Can you work these out from the model? Positions are in its coordinate system, mm. Round coordinates to 2 decimals unless told otherwise and drop trailing zeros. Order: outer loops, then holes, each group sorted by start corner. A loop starts at its lowest first (then second) coordinate and runs counter-clockwise, first axis right, second up. Notation, with made-up numbers: M 9,18.25 L 34,18.25 A18 ccw 34,46.25 Z; hole C 43,57 d2. An arc over 180 degrees is marked long. Answer as CSV lines item,"result". Start each with the question number.
from build123d import *

# Parameters (mm, degrees)
SKETCH10_R         = 15
CUT_EXTRUDE1_DEPTH = 31
SKETCH11_R         = 25
CUT_EXTRUDE2_DEPTH = 31


with BuildPart() as part:
    # Sketch6 → Revolve3 (revolve)
    with BuildSketch(Plane(origin=(0, 0, 0), x_dir=(1, 0, 0), z_dir=(0, 1, 0))):
        with BuildLine():
            Line((-1.369e-06, 75.786874096), (109.999998631, 75.786874096))
            ThreePointArc((109.999998631, 75.786874096), (124.999998631, 60.786874096), (109.999998631, 45.786874096))
            Line((109.999998631, 45.786874096), (-1.369e-06, 45.786874096))
            Line((-1.369e-06, 45.786874096), (-1.369e-06, 75.786874096))
        make_face()
    revolve(axis=Axis((-1.369e-06, 0, -75.786874096), (0, 0, 1)))

    # Sketch10 → Cut-Extrude1 (cut, through all)
    with BuildSketch(Plane.XY.offset(-45.786874096)):
        Circle(SKETCH10_R)
    extrude(amount=-CUT_EXTRUDE1_DEPTH, mode=Mode.SUBTRACT)

    # Sketch11 → Cut-Extrude2 (cut, through all)
    with BuildSketch(Plane.XY.offset(-45.786874096)):
        with Locations((0, 61.701118812)):
            Circle(SKETCH11_R)
        with Locations((61.701118812, 0)):
            Circle(SKETCH11_R)
        with Locations((0, -61.701118812)):
            Circle(SKETCH11_R)
        with Locations((-61.701118812, 0)):
            Circle(SKETCH11_R)
    extrude(amount=-CUT_EXTRUDE2_DEPTH, mode=Mode.SUBTRACT)


solid = part.part
(1) I want a section at C-C on x = 0. Count the separate pieces of the cut face and the enclosed holes in it, and give its area (3 significant figures).
(2) I want a section at B-B on z = -54. Write out the boundary of the cut face in (x, y).
(3) If I drill on line 1 along Y through (x, z) = (0, -60.5); line 2 along Y through (x, z) = (0, -57); line 3 along X through (y, z) = (9.5, -65.5), over which ranges is the centre line in solid material (lowest first)?
(4) I'm going to push flat-ended pins straight in: P1, Ø4, axis at y = -22.5, z = -52.5, coming from the +X side; P2, Ø1.5, axis at y = 0, z = -62.5, coming from the +X side; P3, Ø12, axis at x = 61.5, z = -67, coming from the -Y side. Where does each tip first touch, or does it pass through?
(5) I want a section at A-A on y = 0. Write out the boundary of the cut face in (x, z), and give its area (3 significant figures).
(6) If we mould it in two halves opening along Y, with no side actions, what happens to faces 1 (the cylindrical face through (-3.25, 86.49, -60.58)), 2 (the flat face through (23, 2, -45.787)), 3 (the cylindrical face through (-14.985, 0.66, -60.577))? For each: +Y half, -Y half, draft (parallel to the pull), parting line (faces both ways), or undercut.
From the geometry:
1,separate pieces,"4"
1,enclosed holes,"0"
1,area,"3,410 mm²"
2,outline,"C 0,0 d246.75; hole C -61.7,0 d50; hole C 0,-61.7 d50; hole C 0,61.7 d50; hole C 0,0 d30; hole C 61.7,0 d50"
3,line 1,"-125 to -86.7, -36.7 to -15, 15 to 36.7, 86.7 to 125"
3,line 2,"-124.51 to -86.7, -36.7 to -15, 15 to 36.7, 86.7 to 124.51"
3,line 3,"-123.88 to -84.83, -38.58 to -11.61, 11.61 to 38.58, 84.83 to 123.88"
4,P1,"x = 121.62"
4,P2,"x = 124.97"
4,P3,"y = -111.22"
5,outline,"M -110,-75.79 L -86.7,-75.79 L -86.7,-45.79 L -110,-45.79 A15 ccw Z; M -36.7,-75.79 L -15,-75.79 L -15,-45.79 L -36.7,-45.79 Z; M 15,-75.79 L 36.7,-75.79 L 36.7,-45.79 L 15,-45.79 Z; M 86.7,-75.79 L 110,-75.79 A15 ccw 110,-45.79 L 86.7,-45.79 Z"
5,area,"3,410 mm²"
6,face 1,"undercut"
6,face 2,"draft"
6,face 3,"undercut"
